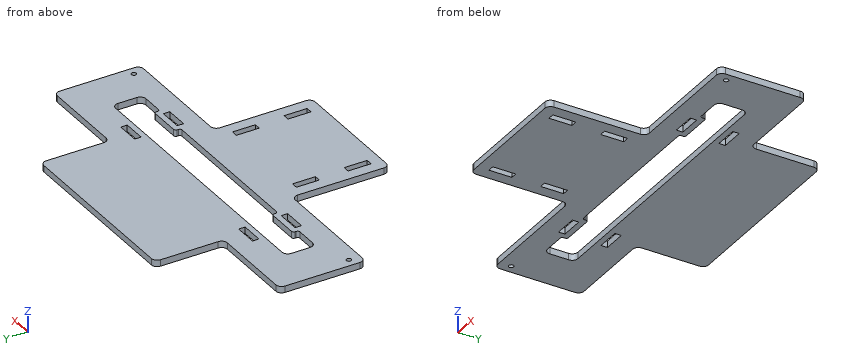
from build123d import *

# Parameters (mm, degrees)
SKETCH_1_W          = 325
SKETCH_1_H          = 230
SKETCH_1_R          = 2.1
EXTRUDE_1_DEPTH     = 5.6
SKETCH_2_W          = 5.6
SKETCH_2_H          = 20
SKETCH_2_W_2        = 20
SKETCH_2_H_2        = 5.6
CUT_EXTRUDE_1_DEPTH = 200.154738834
SKETCH_3_R          = 2.1
SKETCH_3_W          = 56.1
SKETCH_3_H          = 10
CUT_EXTRUDE_2_DEPTH = 200.154738834
CUT_EXTRUDE_3_DEPTH = 200.154738834
SKETCH_5_W          = 80
SKETCH_5_H          = 60
CUT_EXTRUDE_4_DEPTH = 200.154738834
FILLET_1_R          = 5
FILLET_2_R          = 2


with BuildPart() as part:
    # ｽｹｯﾁ1 → ﾎﾞｽ - 押し出し1 (new body)
    with BuildSketch(Plane.XY):
        Rectangle(SKETCH_1_W, SKETCH_1_H)
        with Locations((155, 110)):
            Circle(SKETCH_1_R, mode=Mode.SUBTRACT)
        with Locations(Location((155, -110, 0), (0, 0, 180))):
            Circle(SKETCH_1_R, mode=Mode.SUBTRACT)
        with Locations(Location((-155, 110, 0), (0, 0, 180))):
            Circle(SKETCH_1_R, mode=Mode.SUBTRACT)
        with Locations((-155, -110)):
            Circle(SKETCH_1_R, mode=Mode.SUBTRACT)
        with Locations((155, -10)):
            Circle(SKETCH_1_R, mode=Mode.SUBTRACT)
        with Locations(Location((-155, -10, 0), (0, 0, 180))):
            Circle(SKETCH_1_R, mode=Mode.SUBTRACT)
    extrude(amount=EXTRUDE_1_DEPTH)

    # ｽｹｯﾁ2 → ｶｯﾄ - 押し出し1 (cut, through all)
    with BuildSketch(Plane.XY.offset(5.6)):
        with Locations((43.3, -40)):
            Rectangle(SKETCH_2_W, SKETCH_2_H)
        with Locations((-43.3, -40)):
            Rectangle(SKETCH_2_W, SKETCH_2_H)
        with Locations((43.3, -85)):
            Rectangle(SKETCH_2_W, SKETCH_2_H)
        with Locations((-43.3, -85)):
            Rectangle(SKETCH_2_W, SKETCH_2_H)
        with Locations((85, -2.2)):
            Rectangle(SKETCH_2_W_2, SKETCH_2_H_2)
        with Locations((-85, -2.2)):
            Rectangle(SKETCH_2_W_2, SKETCH_2_H_2)
        with Locations((85, 34.8)):
            Rectangle(SKETCH_2_W_2, SKETCH_2_H_2)
        with Locations((-85, 34.8)):
            Rectangle(SKETCH_2_W_2, SKETCH_2_H_2)
    extrude(amount=-CUT_EXTRUDE_1_DEPTH, mode=Mode.SUBTRACT)

    # ｽｹｯﾁ3 → ｶｯﾄ - 押し出し2 (cut, through all)
    # profile 1 of 4: a face of its own
    with BuildSketch(Plane.XY.offset(5.6)):
        Polygon((-56.1, -115), (-56.1, -105), (-56.1, -20), (-162.5, -20), (-162.5, -115), align=None)
        with Locations((-155, -110)):
            Circle(SKETCH_3_R, mode=Mode.SUBTRACT)
    # profile 2 of 4: a face of its own
    with BuildSketch(Plane.XY.offset(5.6)):
        with Locations((-28.05, -110)):
            Rectangle(SKETCH_3_W, SKETCH_3_H)
    # profile 3 of 4: a face of its own
    with BuildSketch(Plane.XY.offset(5.6)):
        with Locations((28.05, -110)):
            Rectangle(SKETCH_3_W, SKETCH_3_H)
    # profile 4 of 4: a face of its own
    with BuildSketch(Plane.XY.offset(5.6)):
        Polygon((56.1, -20), (56.1, -105), (56.1, -115), (162.5, -115), (162.5, -20), align=None)
        with Locations((155, -110)):
            Circle(SKETCH_3_R, mode=Mode.SUBTRACT)
    extrude(amount=-CUT_EXTRUDE_2_DEPTH, mode=Mode.SUBTRACT)

    # ｽｹｯﾁ4 → ｶｯﾄ - 押し出し3 (cut, through all)
    with BuildSketch(Plane.XY.offset(5.6)):
        Polygon((-125, 27), (125, 27), (125, 5.6), (125, 0.6), (100, 0.6), (100, 5.6), (70, 5.6), (70, 0.6), (-70, 0.6), (-70, 5.6), (-100, 5.6), (-100, 0.6), (-125, 0.6), (-125, 5.6), align=None)
    extrude(amount=-CUT_EXTRUDE_3_DEPTH, mode=Mode.SUBTRACT)

    # ｽｹｯﾁ5 → ｶｯﾄ - 押し出し4 (cut, through all)
    with BuildSketch(Plane.XY.offset(5.6)):
        with Locations((-122.5, 85)):
            Rectangle(SKETCH_5_W, SKETCH_5_H)
        with Locations((122.5, 85)):
            Rectangle(SKETCH_5_W, SKETCH_5_H)
    extrude(amount=-CUT_EXTRUDE_4_DEPTH, mode=Mode.SUBTRACT)

    # ﾌｨﾚｯﾄ1
    fillet_1_edges = [part.edges().sort_by_distance(p)[0] for p in [
        (-162.5, -20, 2.8),
        (-56.1, -20, 2.8),
        (-56.1, -105, 2.8),
        (56.1, -105, 2.8),
        (56.1, -20, 2.8),
        (162.5, -20, 2.8),
        (125, 0.6, 2.8),
        (-125, 0.6, 2.8),
        (-125, 27, 2.8),
        (125, 27, 2.8),
        (-162.5, 55, 2.8),
        (-82.5, 115, 2.8),
        (-82.5, 55, 2.8),
        (82.5, 115, 2.8),
        (162.5, 55, 2.8),
        (82.5, 55, 2.8),
    ]]
    fillet(fillet_1_edges, radius=FILLET_1_R)

    # ﾌｨﾚｯﾄ2
    fillet_2_edges = [part.edges().sort_by_distance(p)[0] for p in [
        (100, 0.6, 2.8),
        (100, 5.6, 2.8),
        (70, 5.6, 2.8),
        (70, 0.6, 2.8),
        (-70, 0.6, 2.8),
        (-70, 5.6, 2.8),
        (-100, 5.6, 2.8),
        (-100, 0.6, 2.8),
    ]]
    fillet(fillet_2_edges, radius=FILLET_2_R)


solid = part.part
Geometry: final body of the model. Coordinates: model frame, mm. Round coordinates to 2 decimals unless told otherwise and drop trailing zeros. Loops run counter-clockwise (first coordinate to the right, second up) from the corner with the lowest first, then second, coordinate; pieces in that order, holes last. Notation, with made-up numbers: M 0,70.25 L 54,70.25 A17 ccw 54,84.25 Z; hole C 16,37.25 d3. An arc over 180 degrees is marked long. Put each result on its own line as item: value. Start each with the question number.
(1) Material intervals for line 1 along X through (y, z) = (-36, 1.1); line 2 along Y through (x, z) = (-87.5, 3.15); line 3 along Y through (x, z) = (-45, 3.2), sorted ascending. Write a range as [from, to].
(2) Section query D-D (y = 88.5). Return loops of the section in (x, z), then the cut area to 3 significant figures.
(3) Section query C-C (x = 131). Return loops of the section in (y, z), then the cut area to 3 significant figures.
(4) Section query A-A (y = -79.5). Return loops of the section in (x, z).
(5) Contact query for flat-ended pins moving along their axis: pin 1 Ø3 at (y, z) = (-65.5, 3.5) entering from +X; pin 2 Ø4 at (x, y) = (-155, -10) entering from -Z; pin 3 Ø3 at (x, z) = (-83, 3.5) entering from -Y; pin 4 Ø1.7 at (x, z) = (-89.5, 3.5) entering from +Y. Output: stop coordinate, or through.
(6) Section query B-B (z = 4.45). State how many separate pieces and enclosed holes the cut face has, then the cut area to 3 significant figures.
Findings below:
1. line 1: x = [-56.1, -46.1], [-40.5, 40.5], [46.1, 56.1]
1. line 2: y = [-20, -5], [0.6, 5.6], [27, 32], [37.6, 55]
1. line 3: y = [-105, -95], [-75, -50], [-30, 0.6], [27, 115]
2. outline: M -82.5,0 L 82.5,0 L 82.5,5.6 L -82.5,5.6 Z
2. area: 924 mm2
3. outline: M -20,0 L 55,0 L 55,5.6 L -20,5.6 Z
3. area: 420 mm2
4. outline: M -56.1,0 L -46.1,0 L -46.1,5.6 L -56.1,5.6 Z; M -40.5,0 L 40.5,0 L 40.5,5.6 L -40.5,5.6 Z; M 46.1,0 L 56.1,0 L 56.1,5.6 L 46.1,5.6 Z
5. pin 1: stops at x = 56.1
5. pin 2: passes through
5. pin 3: stops at y = -20
5. pin 4: stops at y = 55
6. separate pieces: 1
6. enclosed holes: 11
6. area: 36,600 mm2
